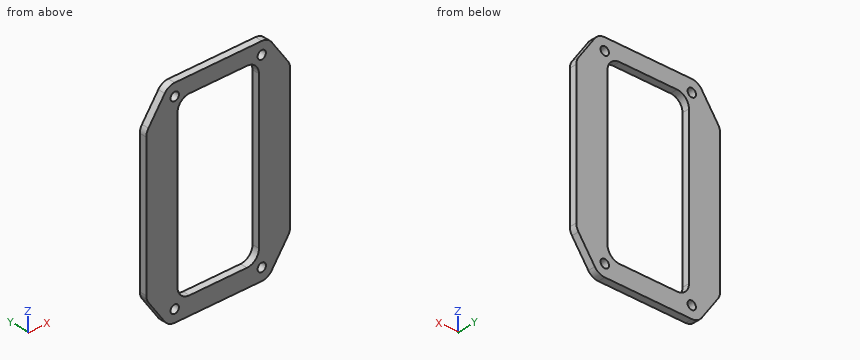
```python
from build123d import *

# Parameters (mm, degrees)
SKETCH1_W           = 60
SKETCH1_H           = 88
SKETCH1_R           = 1.75
SKETCH1_W_2         = 34
SKETCH1_H_2         = 74
BOSS_EXTRUDE1_DEPTH = 3
FILLET1_R           = 5
SKETCH6_W           = 62
SKETCH6_H           = 90
CUT_EXTRUDE3_DEPTH  = 4
FILLET3_R           = 5.05


with BuildPart() as part:
    # Sketch1 → Boss-Extrude1 (new body)
    with BuildSketch(Plane(origin=(0, 0, 0), x_dir=(1, 0, 0), z_dir=(0, 1, 0))):
        with Locations((30, 44)):
            Rectangle(SKETCH1_W, SKETCH1_H)
        with Locations((11.85, 82.95)):
            Circle(SKETCH1_R, mode=Mode.SUBTRACT)
        with Locations((48.15, 82.95)):
            Circle(SKETCH1_R, mode=Mode.SUBTRACT)
        with Locations((48.15, 5.05)):
            Circle(SKETCH1_R, mode=Mode.SUBTRACT)
        with Locations((11.85, 5.05)):
            Circle(SKETCH1_R, mode=Mode.SUBTRACT)
        with Locations((30, 43.5)):
            Rectangle(SKETCH1_W_2, SKETCH1_H_2, mode=Mode.SUBTRACT)
    extrude(amount=BOSS_EXTRUDE1_DEPTH)

    # Fillet1
    fillet1_edges = [part.edges().sort_by_distance(p)[0] for p in [
        (13, 1.5, -80.5),
        (13, 1.5, -6.5),
        (47, 1.5, -6.5),
        (47, 1.5, -80.5),
    ]]
    fillet(fillet1_edges, radius=FILLET1_R)

    # Sketch6 → Cut-Extrude3 (cut, through all)
    with BuildSketch(Plane(origin=(0, 3, 0), x_dir=(1, 0, 0), z_dir=(0, 1, 0))):
        with Locations((30, 44)):
            Rectangle(SKETCH6_W, SKETCH6_H)
        Polygon((9.196567368, 88), (0, 74.65), (0, 13.35), (9.196567368, 0), (50.803432632, 0), (60, 13.35), (60, 74.65), (50.803432632, 88), align=None, mode=Mode.SUBTRACT)
    extrude(amount=-CUT_EXTRUDE3_DEPTH, mode=Mode.SUBTRACT)

    # Fillet3
    fillet3_edges = [part.edges().sort_by_distance(p)[0] for p in [
        (0, 1.5, -74.65),
        (9.196567368, 1.5, -88),
        (50.803432632, 1.5, -88),
        (60, 1.5, -74.65),
        (60, 1.5, -13.35),
        (50.803432632, 1.5, 0),
        (9.196567368, 1.5, 0),
        (0, 1.5, -13.35),
    ]]
    fillet(fillet3_edges, radius=FILLET3_R)


solid = part.part
```
Can you work these out from the model? Positions are in its coordinate system, mm. Give positions to 0.01 mm unless a question says otherwise; leave off trailing zeros. Write each loop counter-clockwise with the first axis right and the second up, starting at its lowest first coordinate (ties: lowest second). Pieces come first, ordered by that corner, then holes. Notation, with made-up numbers: (60.5, 13) - (78.5, 13) arc R12 ccw to (78.5, 20) - close; hole circle Ø5 at (-14.5, -21). An arc over 180 degrees is marked (long way). Write item = value, one per line. Start each with the question number.
1. Imagine slicing it at B-B (y = 2.1). Please give me the cut outline in (x, z).
2. Please list where these lines run through material, in increasing order: line 1 (Z direction, x = 12, y = 1.65); line 2 (Z direction, x = 30, y = 2.95); line 3 (X direction, y = 1.05, z = -5.05).
3. Imagine slicing it at A-A (x = 45). Please give me the cut outline in (y, z).
4. Imagine slicing it at D-D (z = -82.95). Please give me the cut outline in (x, y).
5. Imagine slicing it at C-C (z = -16). Please give me the cut outline in (x, y).
Worked answers:
q1.outline = (0, -73.08) arc R5.05 ccw to (0.89, -75.94) - (7.69, -85.81) arc R5.05 ccw to (11.85, -88) - (48.15, -88) arc R5.05 ccw to (52.31, -85.81) - (59.11, -75.94) arc R5.05 ccw to (60, -73.08) - (60, -14.92) arc R5.05 ccw to (59.11, -12.06) - (52.31, -2.19) arc R5.05 ccw to (48.15, 0) - (11.85, 0) arc R5.05 ccw to (7.69, -2.19) - (0.89, -12.06) arc R5.05 ccw to (0, -14.92) - close; hole circle Ø3.5 at (11.85, -82.95); hole circle Ø3.5 at (11.85, -5.05); hole (13, -75.5) arc R5 ccw to (18, -80.5) - (42, -80.5) arc R5 ccw to (47, -75.5) - (47, -11.5) arc R5 ccw to (42, -6.5) - (18, -6.5) arc R5 ccw to (13, -11.5) - close; hole circle Ø3.5 at (48.15, -82.95); hole circle Ø3.5 at (48.15, -5.05)
q2.line_1 = -88 to -84.69, -81.21 to -6.79, -3.31 to 0
q2.line_2 = -88 to -80.5, -6.5 to 0
q2.line_3 = 5.72 to 10.1, 13.6 to 46.4, 49.9 to 54.28
q3.outline = (0, -88) - (3, -88) - (3, -79.5) - (0, -79.5) - close; (0, -7.5) - (3, -7.5) - (3, 0) - (0, 0) - close
q4.outline = (5.72, 0) - (10.1, 0) - (10.1, 3) - (5.72, 3) - close; (13.6, 0) - (46.4, 0) - (46.4, 3) - (13.6, 3) - close; (49.9, 0) - (54.28, 0) - (54.28, 3) - (49.9, 3) - close
q5.outline = (0, 0) - (13, 0) - (13, 3) - (0, 3) - close; (47, 0) - (60, 0) - (60, 3) - (47, 3) - close
